Source: CAD feature listing. Evaluate the final solid. Frame: model axes, mm. A direction names the side the tool comes from. Give positions to 0.01 mm unless a question says otherwise; leave off trailing zeros. Order: outer loops, then holes, each group sorted by start corner. A loop starts at its lowest first (then second) coordinate and runs counter-clockwise, first axis right, second up.
1) Access query for faces 1 (the face through (72, 0, 177.8)), 2 (the face through (-156, -60, 177.8)), 3 (the face through (-180.246, 63.378, 182.629)). Directions: +Z, -Z, +X, -X, +Y, -Y. A direction counts if a zero-diameter tool reaches every point of the face in a straight line with its end or side. Return the directions, or none.
2) Draft query along Y for faces 4 (the face through (-118, -69.056, 183)), 5 (the face through (-156, -95.25, 182)), 6 (the face through (226, 0, 0)). Return one class per face: released by +Y, released by -Y, zero draft, split by the parting line, or undercut.
3) Section D-D, the plane x = 98. Return loops of the section in (y, z), plus the area to 3 significant figures.
4) Section C-C, the plane z = 113.5. Return loops of the section in (x, y) (3 decimals).
5) Section A-A, the plane y = 52. Return loops of the section in (x, z) (3 decimals), plus the area to 3 significant figures.
6) First-contact query: P1, Ø10, axis at x = -150.5, z = 104, coming from the -Y side; P2, Ø12, axis at x = 48.5, z = 98, coming from the +Y side; P3, Ø17.5, axis at x = 80, y = 3.5, coming from the +Z side; P4, Ø13, axis at x = 203.962, y = 66.548, coming from the +Z side. Flat tips, straight axial feed; report the tip coordinate or a pass-through.
7) Section B-B, the plane x = -4.5. Return loops of the section in (y, z).
8) Material intervals for line 1 (Z direction, x = 11, y = 7); line 2 (Z direction, x = -110, y = 17.5) (3 decimals); line 3 (Z direction, x = -131, y = -76) (3 decimals), sorted ascending.
```python
from build123d import *

# Parameters (mm, degrees)
F1_DEPTH  = 231.775
F3_W      = 165.1
F3_H      = 9.652
F4_DEPTH  = 158.75
F6_D      = 14.2875
F9_DEPTH  = 63.5
F11_DEPTH = 196.978
F12_SIZE  = 88.9


with BuildPart() as f1:
    # F0 (on Right) → F1 (new body, symmetric)
    with BuildSketch(Plane.YZ):
        with BuildLine():
            Line((-26.543, 177.8), (-26.543, 0))
            Line((-26.543, 0), (0, 0))
            Line((0, 0), (0, 9.144))
            Line((0, 9.144), (-14.859, 9.144))
            ThreePointArc((-14.859, 9.144), (-19.3491280605, 11.0038719395), (-21.209, 15.494))
            Line((-21.209, 15.494), (-21.209, 162.306))
            ThreePointArc((-21.209, 162.306), (-19.3491280605, 166.7961280605), (-14.859, 168.656))
            Line((-14.859, 168.656), (0, 168.656))
            Line((0, 168.656), (0, 177.8))
            Line((0, 177.8), (-26.543, 177.8))
        make_face()
        with BuildLine():
            Line((0, 9.144), (0, 0))
            Line((0, 0), (26.543, 0))
            Line((26.543, 0), (26.543, 2.794))
            ThreePointArc((26.543, 2.794), (24.6831280605, 7.2841280605), (20.193, 9.144))
            Line((20.193, 9.144), (0, 9.144))
        make_face()
        with BuildLine():
            Line((26.543, 177.8), (0, 177.8))
            Line((0, 177.8), (0, 168.656))
            Line((0, 168.656), (20.193, 168.656))
            ThreePointArc((20.193, 168.656), (24.6831280605, 170.5158719395), (26.543, 175.006))
            Line((26.543, 175.006), (26.543, 177.8))
        make_face()
    extrude(amount=F1_DEPTH, both=True)

    # F3 (on offset) → F4 (join)
    with BuildSketch(Plane.YZ.offset(219.837)):
        with Locations((0, -4.826)):
            Rectangle(F3_W, F3_H)
    extrude(amount=-F4_DEPTH)

    # F6 (through all)
    with Locations(Plane(origin=(0, 0, -9.652), x_dir=(1, 0, 0), z_dir=(0, 0, -1))):
        with Locations((203.962, -66.548), (76.962, -66.548), (203.962, 66.548), (76.962, 66.548)):
            Hole(F6_D / 2)

    # F8 (on offset) → F9 (join, symmetric)
    with BuildSketch(Plane(origin=(-155.575, 0, 0), x_dir=(0, -1, 0), z_dir=(-1, 0, 0))):
        Polygon((-95.25, 177.8), (26.543, 177.8), (95.25, 177.8), (95.25, 187.325), (-95.25, 187.325), align=None)
    extrude(amount=F9_DEPTH, both=True)

    # F10 (on face) → F11 (cut, through all)
    with BuildSketch(Plane.XY.offset(187.325)):
        with BuildLine():
            ThreePointArc((-185.801, -69.05625), (-180.24475, -63.5), (-185.801, -57.94375))
            Line((-185.801, -57.94375), (-201.549, -57.94375))
            ThreePointArc((-201.549, -57.94375), (-207.10525, -63.5), (-201.549, -69.05625))
            Line((-201.549, -69.05625), (-185.801, -69.05625))
        make_face()
        with BuildLine():
            Line((-109.601, -57.94375), (-125.349, -57.94375))
            ThreePointArc((-125.349, -57.94375), (-130.90525, -63.5), (-125.349, -69.05625))
            Line((-125.349, -69.05625), (-109.601, -69.05625))
            ThreePointArc((-109.601, -69.05625), (-104.04475, -63.5), (-109.601, -57.94375))
        make_face()
        with BuildLine():
            Line((-185.801, 69.05625), (-201.549, 69.05625))
            ThreePointArc((-201.549, 69.05625), (-207.10525, 63.5), (-201.549, 57.94375))
            Line((-201.549, 57.94375), (-185.801, 57.94375))
            ThreePointArc((-185.801, 57.94375), (-180.24475, 63.5), (-185.801, 69.05625))
        make_face()
        with BuildLine():
            ThreePointArc((-125.349, 69.05625), (-130.90525, 63.5), (-125.349, 57.94375))
            Line((-125.349, 57.94375), (-109.601, 57.94375))
            ThreePointArc((-109.601, 57.94375), (-104.04475, 63.5), (-109.601, 69.05625))
            Line((-109.601, 69.05625), (-125.349, 69.05625))
        make_face()
    extrude(amount=-F11_DEPTH, mode=Mode.SUBTRACT)

    # F12
    f12_edges = [f1.edges().sort_by_distance(p)[0] for p in [
        (-231.775, 0, 0),
    ]]
    chamfer(f12_edges, length=F12_SIZE)


solid = f1.part
```
From the geometry:
1. face 1: +Z, +X, +Y, -Y
1. face 2: -Z, +X, -X, -Y
1. face 3: +Z, -Z
2. face 4: undercut
2. face 5: released by -Y
2. face 6: zero draft
3. outline: (-82.55, -9.65) - (82.55, -9.65) - (82.55, 0) - (26.54, 0) - (26.54, 2.79) arc R6.35 ccw to (20.19, 9.14) - (-14.86, 9.14) arc R6.35 cw to (-21.21, 15.49) - (-21.21, 162.31) arc R6.35 cw to (-14.86, 168.66) - (20.19, 168.66) arc R6.35 ccw to (26.54, 175.01) - (26.54, 177.8) - (-26.54, 177.8) - (-26.54, 0) - (-82.55, 0) - close
3. area: 3,420 mm2
4. outline: (-231.775, -26.543) - (231.775, -26.543) - (231.775, -21.209) - (-231.775, -21.209) - close
5. outline: (-219.075, 177.8) - (-92.075, 177.8) - (-92.075, 187.325) - (-219.075, 187.325) - close; (61.087, -9.652) - (219.837, -9.652) - (219.837, 0) - (61.087, 0) - close
5. area: 2,740 mm2
6. P1: stops at y = -26.54
6. P2: stops at y = -21.21
6. P3: stops at z = 177.8
6. P4: passes through
7. outline: (-26.54, 0) - (26.54, 0) - (26.54, 2.79) arc R6.35 ccw to (20.19, 9.14) - (-14.86, 9.14) arc R6.35 cw to (-21.21, 15.49) - (-21.21, 162.31) arc R6.35 cw to (-14.86, 168.66) - (20.19, 168.66) arc R6.35 ccw to (26.54, 175.01) - (26.54, 177.8) - (-26.54, 177.8) - close
8. line 1: z = 0 to 9.14, 168.66 to 177.8
8. line 2: z = 0 to 9.144, 168.656 to 187.325
8. line 3: z = 177.8 to 187.325
